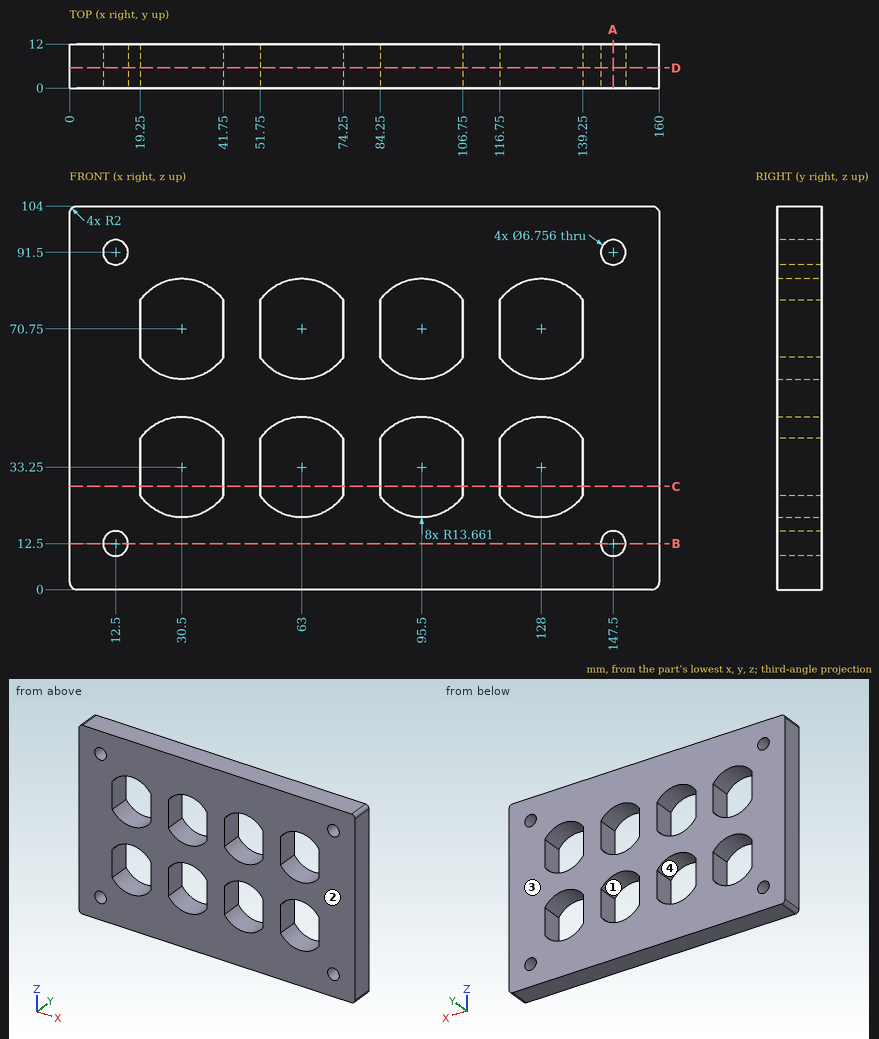
Answer from the drawing. Dimensions are ordinates in mm from the lowest x, y and z of the part. A direction names the side the tool comes from. Coordinates: 2 decimals unless noted, no trailing zeros. Order: outer loops, then holes, each group sorted by start corner. A loop starts at its lowest first (then second) coordinate and runs counter-clockwise, first axis right, second up. Notation, with made-up numbers: M 82,87.5 L 86,87.5 A14 ccw 86,93.5 Z; hole C -18.5,46.25 d4. An arc over 180 degrees is marked long. Put each result on its own line as item: value. Start each with the question number.
Item 1: Consider probe 1 along X at (y, z) = (7.75, 40.5); probe 2 along Z at (x, y) = (147.5, 9.75); probe 3 along X at (y, z) = (8, 12.5). Determine where each line is inside the solid, lowest interval first. Write a range as [from, to].
Item 2: The mould has two halves that part along X. Classify the marked faces 3 and 4: +X half, -X half, draft (parallel to the pull), parting line (faces both ways), or undercut.
Item 3: Given pin 1 Ø2 at (x, z) = (126.5, 21.5) entering from +Y, flat-ended and moving along its own axis, determine where the tip first touches the part or whether it passes through.
Item 4: Section B-B, the plane z = 12.5 is taken. Determine the outline of the cut face in (x, y).
Item 5: For the marked faces 1 and 2, determine the directions among +Z, -Z, +X, -X, +Y, -Y from which every point of the face is accessible in a straight line to the end or side of a thin tool.
Item 6: Section D-D, the plane y = 5.5 is taken. Count the separate pieces of the cut face and the enclosed holes in it, plus the area to 3 significant figures.
Item 7: Section A-A, the plane x = 147.5 is taken. Determine the outline of the cut face in (y, z), plus the area to 3 significant figures.
Item 8: Section C-C, the plane z = 28 is taken. Determine the outline of the cut face in (x, y), plus the area to 3 significant figures.
Computed:
1. probe 1: x = [0, 19.25], [41.75, 51.75], [74.25, 84.25], [106.75, 116.75], [139.25, 160]
1. probe 2: z = [0, 9.12], [15.88, 88.12], [94.88, 104]
1. probe 3: x = [0, 9.12], [15.88, 144.12], [150.88, 160]
2. face 3: draft
2. face 4: undercut
3. pin 1: passes through
4. outline: M 0,0 L 9.12,0 L 9.12,12 L 0,12 Z; M 15.88,0 L 144.12,0 L 144.12,12 L 15.88,12 Z; M 150.88,0 L 160,0 L 160,12 L 150.88,12 Z
5. face 1: +Y, -Y
5. face 2: +Z, -Z, +X, -X, -Y
6. separate pieces: 1
6. enclosed holes: 12
6. area: 12,200 mm2
7. outline: M 0,0 L 12,0 L 12,9.12 L 0,9.12 Z; M 0,15.88 L 12,15.88 L 12,88.12 L 0,88.12 Z; M 0,94.88 L 12,94.88 L 12,104 L 0,104 Z
7. area: 1,090 mm2
8. outline: M 0,0 L 19.25,0 L 19.25,12 L 0,12 Z; M 41.75,0 L 51.75,0 L 51.75,12 L 41.75,12 Z; M 74.25,0 L 84.25,0 L 84.25,12 L 74.25,12 Z; M 106.75,0 L 116.75,0 L 116.75,12 L 106.75,12 Z; M 139.25,0 L 160,0 L 160,12 L 139.25,12 Z
8. area: 840 mm2
